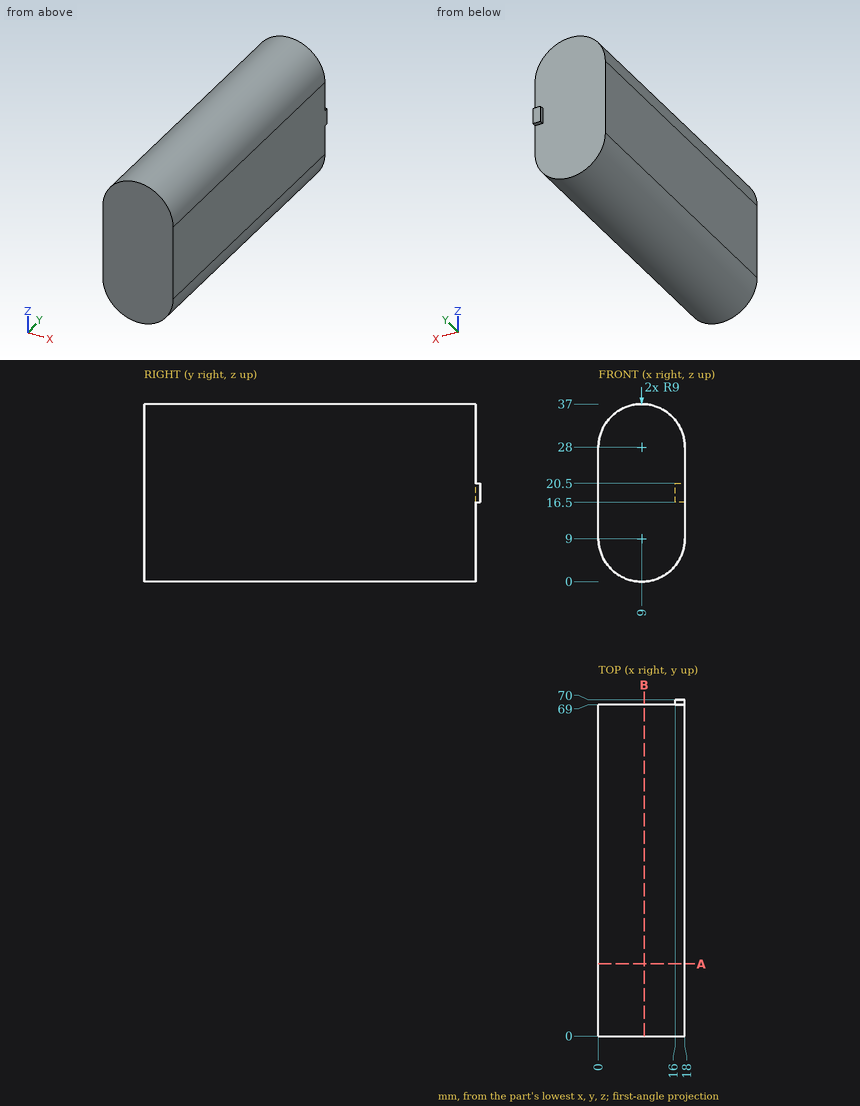
Input: dimensioned drawing with shaded views. Units: mm. Origin: part minimum x, y, z. Coordinates: 2 decimals unless noted, no trailing zeros. Order: outer loops, then holes, each group sorted by start corner. A loop starts at its lowest first (then second) coordinate and runs counter-clockwise, first axis right, second up. Notation, with made-up numbers: (46, -38) - (55, -38) arc R20 ccw to (55, -31) - close; hole circle Ø9 at (89, 1.5). An arc over 180 degrees is marked (long way). Return JSON: item names as keys, results as strings. Group by question number.
1. Material intervals for line 1 along Y through (x, z) = (9.5, 9); line 2 along Z through (x, y) = (7, 46); line 3 along X through (y, z) = (33.5, 31), sorted ascending. Write a range as [from, to].
2. Cut plane A-A (y = 15). Output: boundary loops of the cut face in (x, z), plus the area to 3 significant figures.
3. Cut plane B-B (x = 9.5). Output: boundary loops of the cut face in (y, z), plus the area to 3 significant figures.
4. Pin query (flat end, axial travel): pin 1 (10 mm diameter, centred on x = 8, z = 8.5, fed in from +Y); pin 2 (0.5 mm diameter, centred on y = 69.5, z = 18.5, fed in from -X); pin 3 (0.5 mm diameter, centred on x = 16.5, y = 69.5, fed in from -Z). Return the tip coordinate at first contact, or that it passes through.
Resolved:
{
 "1": {"line 1": "y = [0, 69]", "line 2": "z = [0.23, 36.77]", "line 3": "x = [0.51, 17.49]"},
 "2": {"outline": "(0, 9) arc R9 ccw to (18, 9) - (18, 28) arc R9 ccw to (0, 28) - close", "area": "596 mm²"},
 "3": {"outline": "(0, 0.01) - (69, 0.01) - (69, 36.99) - (0, 36.99) - close", "area": "2,550 mm²"},
 "4": {"pin 1": "stops at y = 69", "pin 2": "stops at x = 16", "pin 3": "stops at z = 16.5"}
}
